```python
from build123d import *

# Parameters (mm, degrees)
F0_W     = 15
F0_H     = 60
F1_DEPTH = 4
F2_W     = 15
F2_H     = 4
F3_DEPTH = 30
F5_ANGLE = -90
F8_R     = 5
F9_R     = 5


with BuildPart() as f1:
    # F0 (on Front) → F1 (new body)
    with BuildSketch(Plane.XZ):
        with Locations((2.568068, 0.993193)):
            Rectangle(F0_W, F0_H)
    extrude(amount=F1_DEPTH)

    # F2 (on face) → F3 (join)
    with BuildSketch(Plane.XZ.offset(4)):
        with Locations((2.568068, 28.993193)):
            Rectangle(F2_W, F2_H)
    extrude(amount=F3_DEPTH)

    # F4 (on face) → F5 (revolve)
    with BuildSketch(Plane(origin=(0, 0, 26.993193), x_dir=(1, 0, 0), z_dir=(0, 0, -1))):
        Polygon((6.068068, 28), (6.068068, 34), (-0.931932, 34), (-0.931932, 28), (1.068068, 28), (1.068068, 24.75), (-0.931932, 24.75), (-0.931932, 12.25), (1.068068, 12.25), (1.068068, 9), (-0.931932, 9), (-0.931932, 4), (6.068068, 4), (6.068068, 9), (4.068068, 9), (4.068068, 12.25), (6.068068, 12.25), (6.068068, 24.75), (4.068068, 24.75), (4.068068, 28), align=None)
    revolve(axis=Axis((2.568068, -4, 26.993193), (-1, 0, 0)), revolution_arc=F5_ANGLE)

    # F8
    f8_edges = [f1.edges().sort_by_distance(p)[0] for p in [
        (2.568068, 0, 30.993193),
    ]]
    fillet(f8_edges, radius=F8_R)

    # F9
    f9_edges = [f1.edges().sort_by_distance(p)[0] for p in [
        (10.068068, -2, -29.006807),
        (-4.931932, -2, -29.006807),
    ]]
    fillet(f9_edges, radius=F9_R)


solid = f1.part
```
For this review, take the finished solid that the model builds, in its own axes (mm). A direction names the side the tool comes from. Round coordinates to 2 decimals unless told otherwise and drop trailing zeros. Write each loop counter-clockwise with the first axis right and the second up, starting at its lowest first coordinate (ties: lowest second). Pieces come first, ordered by that corner, then holes.
1) Take a section at A-A on x = 3. Give the boundary of the cut face in (y, z).
Answer below:
outline: (-34, 26.99) arc R30 ccw to (-4, -3.01) - (-4, -29.01) - (0, -29.01) - (0, 25.99) arc R5 ccw to (-5, 30.99) - (-34, 30.99) - close
2) For line 1 along Z through (x, y) = (4.5, -4.5); line 2 along Z through (x, y) = (9.25, -8); line 3 along X through (y, z) = (-12.5, 15), list the stretches that pass through material, from the lowest coordinate up.
Answer below:
line 1: z = -3 to 3, 6.25 to 18.76, 22.02 to 30.97
line 2: z = 26.99 to 30.99
line 3: x = -0.93 to 6.07
3) Take a section at D-D on y = -13.5. Give the boundary of the cut face in (x, z).
Answer below:
outline: (-4.93, 26.99) - (-0.93, 26.99) - (-0.93, 8.55) - (1.07, 8.55) - (1.07, 4.95) - (-0.93, 4.95) - (-0.93, -1.46) - (6.07, -1.46) - (6.07, 4.95) - (4.07, 4.95) - (4.07, 8.55) - (6.07, 8.55) - (6.07, 26.99) - (10.07, 26.99) - (10.07, 30.99) - (-4.93, 30.99) - close
4) Take a section at C-C on z = 2. Give the boundary of the cut face in (x, y), then the cut area to 3 significant figures.
Answer below:
outline: (-4.93, -4) - (-0.93, -4) - (-0.93, -20.59) - (6.07, -20.59) - (6.07, -4) - (10.07, -4) - (10.07, 0) - (-4.93, 0) - close
area: 176 mm2
5) Insertion check: pin 1 Ø6 at (y, z) = (-9.5, 20.5) entering from +X; pin 2 Ø4 at (y, z) = (-9, 22) entering from -X; pin 3 Ø8 at (x, y) = (1, -24) entering from -Z. Each pin has a flat end and moves straight along its axis. Give the tip position at first contact, or say it passes through.
Answer below:
pin 1: stops at x = 6.07
pin 2: stops at x = -0.93
pin 3: stops at z = 1.62
6) Take a section at B-B on y = -6. Give the boundary of the cut face in (x, z), then the cut area to 3 significant figures.
Answer below:
outline: (-4.93, 26.99) - (-0.93, 26.99) - (-0.93, 22.41) - (1.07, 22.41) - (1.07, 18.99) - (-0.93, 18.99) - (-0.93, 6.34) - (1.07, 6.34) - (1.07, 3.08) - (-0.93, 3.08) - (-0.93, -2.94) - (6.07, -2.94) - (6.07, 3.08) - (4.07, 3.08) - (4.07, 6.34) - (6.07, 6.34) - (6.07, 18.99) - (4.07, 18.99) - (4.07, 22.41) - (6.07, 22.41) - (6.07, 26.99) - (10.07, 26.99) - (10.07, 30.99) - (-4.93, 30.99) - close
area: 243 mm2
7) Machinability: for faces 1 (the face through (1.068, -19, 11)), 2 (the face through (-0.932, -6, 25)), 3 (the face through (6.068, -6, 25)), which of the approach directions +Z, -Z, +X, -X, +Y, -Y give a long, thin tool a straight path to every point of the face, cutting with its end or side? Answer none if there is none.
Answer below:
face 1: -X
face 2: -Z, -X, -Y
face 3: -Z, +X, -Y
8) Mouldability with a two-part tool opening along Z and no side actions: class faces 4 (the face through (6.068, -21, 9)), 5 (the face through (5.082, -21.156, 10.21)), 6 (the face through (2, -19, 30.993)), 7 (the face through (4.068, -8, 23)) as +Z half, -Z half, draft (parallel to the pull), parting line (faces both ways), or undercut.
Answer below:
face 4: draft
face 5: undercut
face 6: +Z half
face 7: undercut
